Check sheet for the modelled part. Datum: model origin and axes. Units: mm. A direction names the side the tool comes from. Round coordinates to 2 decimals unless told otherwise and drop trailing zeros. Order: outer loops, then holes, each group sorted by start corner. A loop starts at its lowest first (then second) coordinate and runs counter-clockwise, first axis right, second up. Notation, with made-up numbers: (9, -9) -> (62, -9) arc R20 ccw to (62, 6) -> close; hole circle Ø10 at (34, -29). An arc over 180 degrees is marked (long way). Answer in a Markdown table with one row per item.
```python
from build123d import *

# Parameters (mm, degrees)
SKETCH1_W           = 24
SKETCH1_H           = 24
BOSS_EXTRUDE1_DEPTH = 6
SKETCH2_W           = 24
SKETCH2_H           = 6
BOSS_EXTRUDE2_DEPTH = 30
SKETCH3_W           = 24
SKETCH3_H           = 6
BOSS_EXTRUDE3_DEPTH = 6
SKETCH4_W           = 24
SKETCH4_H           = 6
BOSS_EXTRUDE4_DEPTH = 6
SKETCH5_W           = 10
SKETCH5_H           = 6
BOSS_EXTRUDE5_DEPTH = 8
FILLET1_R           = 5
FILLET2_R           = 2
FILLET3_R           = 2
SKETCH6_W           = 10
SKETCH6_H           = 6
BOSS_EXTRUDE6_DEPTH = 8
FILLET4_R           = 5
FILLET5_R           = 2
SKETCH7_R           = 1.775
CUT_EXTRUDE1_DEPTH  = 42.568724431
SKETCH8_W           = 6
SKETCH8_H           = 6
BOSS_EXTRUDE7_DEPTH = 2
SKETCH10_W          = 6
SKETCH10_H          = 6
BOSS_EXTRUDE8_DEPTH = 14
BOSS_EXTRUDE9_DEPTH = 50
SKETCH12_R          = 1.905
CUT_EXTRUDE2_DEPTH  = 70.795111418
CUT_EXTRUDE3_REACH  = 70.468
SKETCH13_R          = 1.75


with BuildPart() as part:
    # Sketch1 → Boss-Extrude1 (new body)
    with BuildSketch(Plane(origin=(0, 0, 0), x_dir=(1, 0, 0), z_dir=(0, 1, 0))):
        with Locations((1.896724894, -0.667948192)):
            Rectangle(SKETCH1_W, SKETCH1_H)
    extrude(amount=BOSS_EXTRUDE1_DEPTH)

    # Sketch2 → Boss-Extrude2 (add)
    with BuildSketch(Plane(origin=(0, 6, 0), x_dir=(1, 0, 0), z_dir=(0, 1, 0))):
        with Locations((1.896724894, -6.462948192)):
            Rectangle(SKETCH2_W, SKETCH2_H)
        with Locations((1.896724894, 5.127051808)):
            Rectangle(SKETCH2_W, SKETCH2_H)
    extrude(amount=BOSS_EXTRUDE2_DEPTH)

    # Sketch3 → Boss-Extrude3 (add)
    with BuildSketch(Plane.XY.offset(12.667948192)):
        with Locations((1.896724894, 3)):
            Rectangle(SKETCH3_W, SKETCH3_H)
    extrude(amount=BOSS_EXTRUDE3_DEPTH)

    # Sketch4 → Boss-Extrude4 (add)
    with BuildSketch(Plane(origin=(0, 0, -11.332051808), x_dir=(-1, 0, 0), z_dir=(0, 0, -1))):
        with Locations((-1.896724894, 3)):
            Rectangle(SKETCH4_W, SKETCH4_H)
    extrude(amount=BOSS_EXTRUDE4_DEPTH)

    # Sketch5 → Boss-Extrude5 (add)
    with BuildSketch(Plane(origin=(13.896724894, 0, 0), x_dir=(0, 0, -1), z_dir=(1, 0, 0))):
        with Locations((-0.667948192, 3)):
            Rectangle(SKETCH5_W, SKETCH5_H)
    extrude(amount=BOSS_EXTRUDE5_DEPTH)

    # Fillet1
    # the kernel refuses this fillet: 5 mm, written as the material it adds along each edge
    with BuildSketch(Plane(origin=(13.896724894, 0, -4.332051808), x_dir=(0, 0, -1), z_dir=(0, 1, 0)), Plane(origin=(13.896724894, 6, 5.667948192), x_dir=(0, 0, 1), z_dir=(0, -1, 0))) as fillet1_piece_1:
        with BuildLine():
            CenterArc((FILLET1_R, -FILLET1_R), FILLET1_R, 90, 90)
            Line((0, -FILLET1_R), (0, 0))
            Line((0, 0), (FILLET1_R, 0))
        make_face()
    extrude(amount=6)

    # Fillet2
    fillet2_edges = [part.edges().sort_by_distance(p)[0] for p in [
        (21.896724894, 3, -4.332051808),
        (21.896724894, 3, 5.667948192),
    ]]
    fillet(fillet2_edges, radius=FILLET2_R)

    # Fillet3
    fillet3_edges = [part.edges().sort_by_distance(p)[0] for p in [
        (-10.103275106, 3, 18.667948192),
        (13.896724894, 3, 18.667948192),
        (13.896724894, 3, -17.332051808),
        (-10.103275106, 3, -17.332051808),
    ]]
    fillet(fillet3_edges, radius=FILLET3_R)

    # Sketch6 → Boss-Extrude6 (add)
    with BuildSketch(Plane.ZY.offset(10.103275106)):
        with Locations((0.667948192, 3)):
            Rectangle(SKETCH6_W, SKETCH6_H)
    extrude(amount=BOSS_EXTRUDE6_DEPTH)

    # Fillet4
    # the kernel refuses this fillet: 5 mm, written as the material it adds along each edge
    with BuildSketch(Plane(origin=(-10.103275106, 6, -4.332051808), x_dir=(0, 0, -1), z_dir=(0, -1, 0)), Plane(origin=(-10.103275106, 0, 5.667948192), x_dir=(0, 0, 1), z_dir=(0, 1, 0))) as fillet4_piece_1:
        with BuildLine():
            CenterArc((FILLET4_R, -FILLET4_R), FILLET4_R, 90, 90)
            Line((0, -FILLET4_R), (0, 0))
            Line((0, 0), (FILLET4_R, 0))
        make_face()
    extrude(amount=6)

    # Fillet5
    fillet5_edges = [part.edges().sort_by_distance(p)[0] for p in [
        (-18.103275106, 3, -4.332051808),
        (-18.103275106, 3, 5.667948192),
    ]]
    fillet(fillet5_edges, radius=FILLET5_R)

    # Sketch7 → Cut-Extrude1 (cut, through all)
    with BuildSketch(Plane(origin=(0, 6, 0), x_dir=(1, 0, 0), z_dir=(0, 1, 0))):
        with Locations(Location((1.896724894, -13.667948192, 0), (0, 0, 270))):
            Circle(SKETCH7_R)
        with Locations(Location((-13.103275106, -0.667948192, 0), (0, 0, 270))):
            Circle(SKETCH7_R)
        with Locations(Location((1.896724894, 12.332051808, 0), (0, 0, 270))):
            Circle(SKETCH7_R)
        with Locations(Location((16.896724894, -0.667948192, 0), (0, 0, 270))):
            Circle(SKETCH7_R)
    extrude(amount=-CUT_EXTRUDE1_DEPTH, mode=Mode.SUBTRACT)

    # Sketch8 → Boss-Extrude7 (add)
    with BuildSketch(Plane(origin=(13.896724894, 0, 0), x_dir=(0, 0, -1), z_dir=(1, 0, 0))):
        with Locations((-13.667948192, 3)):
            Rectangle(SKETCH8_W, SKETCH8_H)
    extrude(amount=BOSS_EXTRUDE7_DEPTH)

    # Sketch10 → Boss-Extrude8 (add, along a direction that is not the sketch's normal)
    with BuildSketch(Plane(origin=(15.896724894, 0, 0), x_dir=(0, 0, -1), z_dir=(1, 0, 0))):
        with Locations((-13.667948192, 3)):
            Rectangle(SKETCH10_W, SKETCH10_H)
    extrude(amount=BOSS_EXTRUDE8_DEPTH, dir=(0.9271838545667885, 0, 0.3746065934159094))

    # Sketch11 → Boss-Extrude9 (add)
    with BuildSketch(Plane(origin=(0, 6, 0), x_dir=(1, 0, 0), z_dir=(0, 1, 0))):
        Polygon((28.877298858, -21.9124405), (15.896724894, -16.667948192), (17.980700006, -11.509928791), (28.877298858, -15.9124405), align=None)
    extrude(amount=BOSS_EXTRUDE9_DEPTH)

    # Sketch12 → Cut-Extrude2 (cut, through all)
    with BuildSketch(Plane(origin=(-3.558475874, 0, 8.807536853), x_dir=(0.9271838545667885, 0, 0.3746065934159093), z_dir=(-0.37460659341590935, 0, 0.9271838545667886))):
        with Locations((27.983109954, 14)):
            Circle(SKETCH12_R)
        with Locations((27.983109954, 51.211)):
            Circle(SKETCH12_R)
    extrude(amount=-CUT_EXTRUDE2_DEPTH, mode=Mode.SUBTRACT)

    # Cut-Extrude3: up to this face of the body (flat: up to its plane)
    cut_extrude3_end = Plane(part.part.faces().sort_by_distance((1.896724894, 21, -8.127051808))[0])
    # Sketch13 → Cut-Extrude3 (cut, up to the picked face)
    with BuildSketch(Plane.XY.offset(9.462948192), mode=Mode.PRIVATE) as cut_extrude3_sk1:
        with Locations((1.896724894, 15)):
            Circle(SKETCH13_R)
    cut_extrude3_tool1 = split(extrude(cut_extrude3_sk1.sketch, amount=-CUT_EXTRUDE3_REACH, mode=Mode.PRIVATE), bisect_by=cut_extrude3_end, keep=Keep.BOTH, mode=Mode.PRIVATE)
    # Sketch13 → Cut-Extrude3 (cut, up to the picked face)
    with BuildSketch(Plane.XY.offset(9.462948192), mode=Mode.PRIVATE) as cut_extrude3_sk2:
        with Locations((1.896724894, 25)):
            Circle(SKETCH13_R)
    cut_extrude3_tool2 = split(extrude(cut_extrude3_sk2.sketch, amount=-CUT_EXTRUDE3_REACH, mode=Mode.PRIVATE), bisect_by=cut_extrude3_end, keep=Keep.BOTH, mode=Mode.PRIVATE)
    add(cut_extrude3_tool1.solids().sort_by(Axis((1.896725, 15, 9.462948), (0, 0, -1)))[0], mode=Mode.SUBTRACT)
    add(cut_extrude3_tool2.solids().sort_by(Axis((1.896725, 25, 9.462948), (0, 0, -1)))[0], mode=Mode.SUBTRACT)


solid = part.part
```
(1) Scan lines: probe 1 along Z at (x, y) = (4, 24); probe 2 along Y at (x, z) = (2, 8); probe 3 along Y at (x, z) = (-3, 8.5). Record each from-to range of solid material in increasing order. Write a range as from..to.
Solutions:
| item | result |
|---|---|
| probe 1 | -8.13..-2.13, 3.46..9.46 |
| probe 2 | 0..13.25, 16.75..23.25, 26.75..36 |
| probe 3 | 0..36 |
(2) Tool access check on faces 1 (the flat face through (-10.103, 3, 14)), 2 (the flat face through (16.92, 30.65, 14.13)), 3 (the flat face through (-10.103, 3, -12)), 4 (the flat face through (13.897, 3, -12)), 5 (the flat face through (2, 21, -8.127)). Record the directions out of +Z, -Z, +X, -X, +Y, -Y that give a thin tool (end or side, any length) a straight path to the whole face; none if there is none.
Solutions:
| item | result |
|---|---|
| face 1 | +Z, -X, +Y, -Y |
| face 2 | -Z, -X, +Y |
| face 3 | -Z, -X, +Y, -Y |
| face 4 | -Z, +X, +Y, -Y |
| face 5 | -Z, +X, -X, +Y |
(3) Section check C-C on y = 25. Record the boundary of the cut face in (x, z).
Solutions:
| item | result |
|---|---|
| outline | (-10.1, -8.13) -> (0.15, -8.13) -> (0.15, -2.13) -> (-10.1, -2.13) -> close; (-10.1, 3.46) -> (0.15, 3.46) -> (0.15, 9.46) -> (-10.1, 9.46) -> close; (3.65, -8.13) -> (13.9, -8.13) -> (13.9, -2.13) -> (3.65, -2.13) -> close; (3.65, 3.46) -> (13.9, 3.46) -> (13.9, 9.46) -> (3.65, 9.46) -> close; (15.9, 16.67) -> (17.98, 11.51) -> (28.88, 15.91) -> (28.88, 21.91) -> close |
(4) Section check A-A on y = 7. Record the boundary of the cut face in (x, z).
Solutions:
| item | result |
|---|---|
| outline | (-10.1, -8.13) -> (13.9, -8.13) -> (13.9, -2.13) -> (-10.1, -2.13) -> close; (-10.1, 3.46) -> (13.9, 3.46) -> (13.9, 9.46) -> (-10.1, 9.46) -> close; (15.9, 16.67) -> (17.98, 11.51) -> (28.88, 15.91) -> (28.88, 21.91) -> close |
(5) Draft check along Z on faces 6 (the cylindrical face through (15.32, 2.96, -5.84)), 7 (the flat face through (2, 3, 18.668)), 8 (the flat face through (2, 21, -2.127)). Enter one of: pulls with the +Z half, pulls with the -Z half, needs draft (parallel to the pull), parting line crosses it, or undercut.
Solutions:
| item | result |
|---|---|
| face 6 | pulls with the -Z half |
| face 7 | pulls with the +Z half |
| face 8 | undercut |
(6) Section check D-D on y = 15. Record the boundary of the cut face in (x, z).
Solutions:
| item | result |
|---|---|
| outline | (-10.1, -8.13) -> (0.15, -8.13) -> (0.15, -2.13) -> (-10.1, -2.13) -> close; (-10.1, 3.46) -> (0.15, 3.46) -> (0.15, 9.46) -> (-10.1, 9.46) -> close; (3.65, -8.13) -> (13.9, -8.13) -> (13.9, -2.13) -> (3.65, -2.13) -> close; (3.65, 3.46) -> (13.9, 3.46) -> (13.9, 9.46) -> (3.65, 9.46) -> close; (15.9, 16.67) -> (17.98, 11.51) -> (22.97, 13.52) -> (20.88, 18.68) -> close; (23.89, 19.9) -> (25.97, 14.74) -> (28.88, 15.91) -> (28.88, 21.91) -> close |
(7) Depth check by flat-ended pin: pin 1 Ø1.1 at (x, y) = (19.5, 3) entering from +Z; pin 2 Ø1 at (x, y) = (-8.5, 8.5) entering from -Z; pin 3 Ø3 at (x, y) = (1.9, 15) entering from +Z; pin 4 Ø7 at (x, y) = (5.5, 20.5) entering from +Z. Enter the tip coordinate at first touch or a pass-through.
Solutions:
| item | result |
|---|---|
| pin 1 | z = 18.35 |
| pin 2 | z = -8.13 |
| pin 3 | through |
| pin 4 | z = 9.46 |
(8) Section check B-B on x = -5.5. Record the boundary of the cut face in (y, z), plus the area to 3 significant figures.
Solutions:
| item | result |
|---|---|
| outline | (0, -17.33) -> (6, -17.33) -> (6, -8.13) -> (36, -8.13) -> (36, -2.13) -> (6, -2.13) -> (6, 3.46) -> (36, 3.46) -> (36, 9.46) -> (6, 9.46) -> (6, 18.67) -> (0, 18.67) -> close |
| area | 576 mm^2 |
